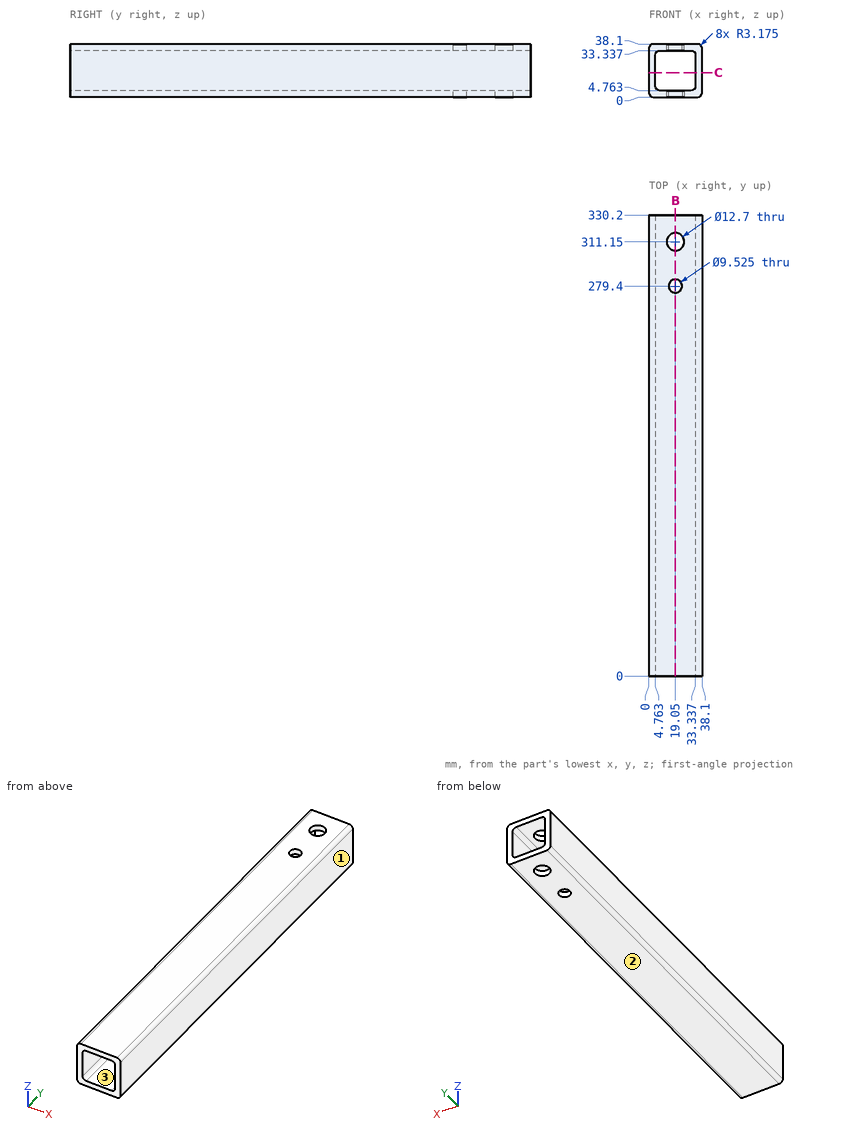
Geometry: see drawing. Coordinates: mm, zero at the bounding-box minimum. Round coordinates to 2 decimals unless told otherwise and drop trailing zeros. Write each loop counter-clockwise with the first axis right and the second up, starting at its lowest first coordinate (ties: lowest second). Pieces come first, ordered by that corner, then holes. Notation, with made-up numbers: (-10, 69.5) -> (33, 69.5) arc R34 cw to (33, 102.5) -> close; hole circle Ø10 at (55, 30). An arc over 180 degrees is marked (long way). Answer as CSV lines item,"result".
1. Contact query for a flat-ended pin moving along its axis: P1, Ø8.5, axis at x = 19.05, y = 279.4, coming from the -Z side. Output: stop coordinate, or through.
Geometry says:
P1,"passes through"
2. Mould query, pull axis Z, two halves, no side actions, for the marked faces 1, 2 and 3. Classes: +Z half, -Z half, draft (parallel to the pull), parting line (faces both ways), or undercut.
Geometry says:
face 1,"draft"
face 2,"-Z half"
face 3,"undercut"
3. Section C-C (z = 17.5). Return the cut outline in (x, y).
Geometry says:
outline,"(0, 0) -> (4.76, 0) -> (4.76, 330.2) -> (0, 330.2) -> close; (33.34, 0) -> (38.1, 0) -> (38.1, 330.2) -> (33.34, 330.2) -> close"
4. Section B-B (x = 19.05). Return the cut outline in (y, z), plus the area to 3 significant figures.
Geometry says:
outline,"(0, 0) -> (274.64, 0) -> (274.64, 4.76) -> (0, 4.76) -> close; (0, 33.34) -> (274.64, 33.34) -> (274.64, 38.1) -> (0, 38.1) -> close; (284.16, 0) -> (304.8, 0) -> (304.8, 4.76) -> (284.16, 4.76) -> close; (284.16, 33.34) -> (304.8, 33.34) -> (304.8, 38.1) -> (284.16, 38.1) -> close; (317.5, 0) -> (330.2, 0) -> (330.2, 4.76) -> (317.5, 4.76) -> close; (317.5, 33.34) -> (330.2, 33.34) -> (330.2, 38.1) -> (317.5, 38.1) -> close"
area,"2,930 mm^2"
5. Ray query, L1, parallel to Y at x = 19, z = 35; L2, parallel to X at y = 279.4, z = 2.6; L3, parallel to Z at x = 30.5, y = 269. Return the intervals inside material, ascending. Write a range as [from, to].
Geometry says:
L1,"y = [0, 274.64], [284.16, 304.8], [317.5, 330.2]"
L2,"x = [0.05, 14.29], [23.81, 38.05]"
L3,"z = [0, 4.78], [33.32, 38.1]"
